from build123d import *

# Parameters (mm, degrees)
F1_DEPTH  = 450
F2_W      = 444
F2_H      = 164.8707569358
F3_DEPTH  = 360.001
F5_DEPTH  = 450.001
F6_W      = 40
F6_H      = 132.1425742267
F7_DEPTH  = 3
F8_R      = 5
F9_R      = 5
F10_R     = 5
F11_R     = 5
F13_DEPTH = 326.2718033332
F15_DEPTH = 25
F16_W     = 415.9923672676
F16_H     = 66.3970857859
F17_DEPTH = 25
F18_W     = 450
F18_H     = 10
F19_DEPTH = 137.8889997614
F20_R     = 5
F21_R     = 5
F22_R     = 5


with BuildPart() as f1:
    # F0 (on Right) → F1 (new body)
    with BuildSketch(Plane.YZ):
        Polygon((0, 0), (0, 360), (-167.8707569358, 0), align=None)
    extrude(amount=F1_DEPTH)

    # F2 (on face) → F3 (cut, through all)
    with BuildSketch(Plane(origin=(0, 0, 0), x_dir=(1, 0, 0), z_dir=(0, 0, -1))):
        with Locations((225, 85.4353784679)):
            Rectangle(F2_W, F2_H)
    extrude(amount=-F3_DEPTH, mode=Mode.SUBTRACT)

    # F4 (on face) → F5 (cut, through all)
    with BuildSketch(Plane(origin=(0, 0, 0), x_dir=(0, -1, 0), z_dir=(-1, 0, 0))):
        Polygon((167.8707569358, 0), (137.8879997614, 64.2982302564), (0, 0), align=None)
    extrude(amount=-F5_DEPTH, mode=Mode.SUBTRACT)

    # F6 (on face) → F7 (join)
    with BuildSketch(Plane(origin=(0, 0, 0), x_dir=(1, 0, 0), z_dir=(0, -0.4226182617, -0.906307787))):
        with Locations((-17, 86.0712871133)):
            Rectangle(F6_W, F6_H)
        with Locations((467, 86.0712871133)):
            Rectangle(F6_W, F6_H)
    extrude(amount=-F7_DEPTH)

    # F8
    f8_edges = [f1.edges().sort_by_distance(p)[0] for p in [
        (-37, -137.254072, 65.657692),
    ]]
    fillet(f8_edges, radius=F8_R)

    # F9
    f9_edges = [f1.edges().sort_by_distance(p)[0] for p in [
        (487, -137.254072, 65.657692),
    ]]
    fillet(f9_edges, radius=F9_R)

    # F10
    f10_edges = [f1.edges().sort_by_distance(p)[0] for p in [
        (487, -17.492228, 9.811827),
    ]]
    fillet(f10_edges, radius=F10_R)

    # F11
    f11_edges = [f1.edges().sort_by_distance(p)[0] for p in [
        (-37, -17.492228, 9.811827),
    ]]
    fillet(f11_edges, radius=F11_R)

    # F12 (on face) → F13 (cut, through all)
    with BuildSketch(Plane(origin=(0, 0, 0), x_dir=(1, 0, 0), z_dir=(0, -0.4226182617, -0.906307787))):
        with BuildLine():
            ThreePointArc((-28.5, 121.0712871133), (-25, 117.5712871133), (-21.5, 121.0712871133))
            Line((-21.5, 121.0712871133), (-21.5, 141.0712871133))
            ThreePointArc((-21.5, 141.0712871133), (-25, 144.5712871133), (-28.5, 141.0712871133))
            Line((-28.5, 141.0712871133), (-28.5, 121.0712871133))
        make_face()
        with BuildLine():
            ThreePointArc((-21.5, 51.0712871133), (-25, 54.5712871133), (-28.5, 51.0712871133))
            Line((-28.5, 51.0712871133), (-28.5, 31.0712871133))
            ThreePointArc((-28.5, 31.0712871133), (-25, 27.5712871133), (-21.5, 31.0712871133))
            Line((-21.5, 31.0712871133), (-21.5, 51.0712871133))
        make_face()
        with BuildLine():
            ThreePointArc((471.5, 121.0712871133), (475, 117.5712871133), (478.5, 121.0712871133))
            Line((478.5, 121.0712871133), (478.5, 141.0712871133))
            ThreePointArc((478.5, 141.0712871133), (475, 144.5712871133), (471.5, 141.0712871133))
            Line((471.5, 141.0712871133), (471.5, 121.0712871133))
        make_face()
        with BuildLine():
            Line((478.5, 31.0712871133), (478.5, 51.0712871133))
            ThreePointArc((478.5, 51.0712871133), (475, 54.5712871133), (471.5, 51.0712871133))
            Line((471.5, 51.0712871133), (471.5, 31.0712871133))
            ThreePointArc((471.5, 31.0712871133), (475, 27.5712871133), (478.5, 31.0712871133))
        make_face()
    extrude(amount=-F13_DEPTH, mode=Mode.SUBTRACT)

    # F14 (on face) → F15 (cut)
    with BuildSketch(Plane(origin=(0, 0, 0), x_dir=(-1, 0, 0), z_dir=(0, 1, 0))):
        with BuildLine():
            ThreePointArc((-428, 307.5), (-425, 304.5), (-422, 307.5))
            Line((-422, 307.5), (-422, 332.5))
            ThreePointArc((-422, 332.5), (-425, 335.5), (-428, 332.5))
            Line((-428, 332.5), (-428, 307.5))
        make_face()
        with BuildLine():
            Line((-28, 332.5), (-28, 307.5))
            ThreePointArc((-28, 307.5), (-25, 304.5), (-22, 307.5))
            Line((-22, 307.5), (-22, 332.5))
            ThreePointArc((-22, 332.5), (-25, 335.5), (-28, 332.5))
        make_face()
        with BuildLine():
            ThreePointArc((-422, 132.5), (-425, 135.5), (-428, 132.5))
            Line((-428, 132.5), (-428, 107.5))
            ThreePointArc((-428, 107.5), (-425, 104.5), (-422, 107.5))
            Line((-422, 107.5), (-422, 132.5))
        make_face()
        with BuildLine():
            ThreePointArc((-22, 132.5), (-25, 135.5), (-28, 132.5))
            Line((-28, 132.5), (-28, 107.5))
            ThreePointArc((-28, 107.5), (-25, 104.5), (-22, 107.5))
            Line((-22, 107.5), (-22, 132.5))
        make_face()
    extrude(amount=-F15_DEPTH, mode=Mode.SUBTRACT)

    # F16 (on face) → F17 (cut)
    with BuildSketch(Plane.XZ.offset(3)):
        with Locations((225, 33.1985428929)):
            Rectangle(F16_W, F16_H)
    extrude(amount=-F17_DEPTH, mode=Mode.SUBTRACT)

    # F18 (on face) → F19 (cut, through all)
    with BuildSketch(Plane(origin=(0, 0, 0), x_dir=(-1, 0, 0), z_dir=(0, 1, 0))):
        with Locations((-225, 355)):
            Rectangle(F18_W, F18_H)
    extrude(amount=-F19_DEPTH, mode=Mode.SUBTRACT)

    # F20
    f20_edges = [f1.edges().sort_by_distance(p)[0] for p in [
        (17.003816, -1.5, 0.699461),
    ]]
    fillet(f20_edges, radius=F20_R)

    # F21
    f21_edges = [f1.edges().sort_by_distance(p)[0] for p in [
        (17.003816, -1.5, 66.397086),
    ]]
    fillet(f21_edges, radius=F21_R)

    # F22
    f22_edges = [f1.edges().sort_by_distance(p)[0] for p in [
        (432.996184, -1.5, 66.397086),
        (432.996184, -1.5, 0.699461),
    ]]
    fillet(f22_edges, radius=F22_R)


solid = f1.part
Build history of the part. All positions in model axes, mm. A direction names the side the tool comes from. Give positions to 0.01 mm unless a question says otherwise; leave off trailing zeros. Loops run counter-clockwise (first coordinate to the right, second up) from the corner with the lowest first, then second, coordinate; pieces in that order, holes last. Notation, with made-up numbers: (16.25, 60.25) -> (53.25, 60.25) arc R28 cw to (53.25, 91.25) -> close; hole circle Ø4 at (20.25, -33). An arc over 180 degrees is marked (long way). Answer in a Markdown table with one row per item.
Item 1: Flat gauge pins, fed straight in: P1, Ø6, axis at x = 193, z = 96.5, coming from the +Y side; P2, Ø3.5, axis at y = -1.5, z = 119, coming from the +X side; P3, Ø0.9, axis at y = -1.5, z = 124, coming from the -X side; P4, Ø4, axis at x = 252, z = 245, coming from the -Y side. Where does each tip first touch, or does it go through?
Findings below:
| item | result |
|---|---|
| P1 | stops at y = 0 |
| P2 | stops at x = 450 |
| P3 | stops at x = 0 |
| P4 | stops at y = -3 |
Item 2: Slice it at B-B on z = 269. Write the cut outline in (x, y).
Findings below:
| item | result |
|---|---|
| outline | (0, -42.43) -> (3, -42.43) -> (3, -3) -> (447, -3) -> (447, -42.43) -> (450, -42.43) -> (450, 0) -> (0, 0) -> close |
Item 3: Tool access for faces 4 (the flat face through (468.241, -77.578, 39.485)), 5 (the flat face through (222, -3, 212)), 6 (the flat face through (-18.759, -77.578, 39.485)), 7 (the flat face through (-37, -77, 37)): list every direction of +Z, -Z, +X, -X, +Y, -Y with a clear straight run to the whole face (end or side of a thin tool).
Findings below:
| item | result |
|---|---|
| face 4 | +Z, +X, +Y |
| face 5 | +Z, -Z, -Y |
| face 6 | +Z, -X, +Y |
| face 7 | +Z, -Z, -X, +Y, -Y |
Item 4: Slice it at A-A on x = 355. Write the cut outline in (y, z).
Findings below:
| item | result |
|---|---|
| outline | (-3, 66.4) -> (0, 66.4) -> (0, 350) -> (-3, 350) -> close |
Item 5: Probe line 1 along X through (y, z) = (-60.5, 77.5); line 2 along Y through (x, z) = (314.5, 299.5). List the from-to ranges inside material, lowest first. Write a range as [from, to].
Findings below:
| item | result |
|---|---|
| line 1 | x = [0, 3], [447, 450] |
| line 2 | y = [-3, 0] |
Item 6: Mould opens along X. For faces 1 (the flat face through (478.5, -118, 57)), 2 (the flat face through (222, 0, 211)), 3 (the flat face through (487, -77, 37)) say: pulls with the +X half, pulls with the -X half, needs draft (parallel to the pull), parting line crosses it, or undercut.
Findings below:
| item | result |
|---|---|
| face 1 | undercut |
| face 2 | needs draft |
| face 3 | pulls with the +X half |
Item 7: Slice it at C-C on z = 210. Write the cut outline in (x, y), plus the area to 3 significant figures.
Findings below:
| item | result |
|---|---|
| outline | (0, -69.95) -> (3, -69.95) -> (3, -3) -> (447, -3) -> (447, -69.95) -> (450, -69.95) -> (450, 0) -> (0, 0) -> close |
| area | 1,750 mm² |
